Design review of the part built by this model. Coordinates are the model's own, in mm. Coordinates: 2 decimals unless noted, no trailing zeros. Write each loop counter-clockwise with the first axis right and the second up, starting at its lowest first coordinate (ties: lowest second). Pieces come first, ordered by that corner, then holes.
```python
from build123d import *

# Parameters (mm, degrees)
EXTRUDE_1_DEPTH = 10


with BuildPart() as part:
    # ｽｹｯﾁ1 → ﾎﾞｽ - 押し出し1 (new body)
    with BuildSketch(Plane(origin=(0, 0, 0), x_dir=(1, 0, 0), z_dir=(0, 1, 0))):
        with BuildLine():
            ThreePointArc((9.1, 0), (10.6, 1.5), (12.1, 0))
            Line((12.1, 0), (25, 0))
            Line((25, 0), (25, 25))
            Line((25, 25), (-25, 25))
            Line((-25, 25), (-25, 0))
            Line((-25, 0), (-15.5, 0))
            ThreePointArc((-15.5, 0), (-14, 1.5), (-12.5, 0))
            Line((-12.5, 0), (0, 0))
            Line((0, 0), (9.1, 0))
        make_face()
        with BuildLine():
            Line((25, 0), (12.1, 0))
            ThreePointArc((12.1, 0), (10.6, -1.5), (9.1, 0))
            Line((9.1, 0), (0, 0))
            Line((0, 0), (-12.5, 0))
            ThreePointArc((-12.5, 0), (-14, -1.5), (-15.5, 0))
            Line((-15.5, 0), (-25, 0))
            Line((-25, 0), (-25, -25))
            Line((-25, -25), (25, -25))
            Line((25, -25), (25, 0))
        make_face()
    extrude(amount=EXTRUDE_1_DEPTH)


solid = part.part
```
(1) Insertion check: pin 1 Ø6 at (x, z) = (20, -10.5) entering from -Y; pin 2 Ø2.5 at (x, z) = (-14, 0) entering from +Y. Each pin has a flat end and moves straight along its axis. Give the tip position at first contact, or say it passes through.
(2) Consider section A-A (x = 10.6). Give the boundary of the cut face in (y, z).
(3) Mouldability with a two-part tool opening along Z and no side actions: class faces 1 (the cylindrical face through (11.986, 4.93, -0.575)), 2 (the flat face through (0, 5, 25)), 3 (the flat face through (0, 5, -25)), 4 (the flat face through (0, 0, 0)) as +Z half, -Z half, draft (parallel to the pull), parting line (faces both ways), or undercut.
(4) Consider section B-B (z = 0). Give the boundary of the cut face in (x, y).
(5) Wall thickness on line 1 (Z direction, x = -14, y = 8.25); line 2 (X direction, y = 3.5, z = -1); line 3 (Z direction, x = 11.5, y = 1.5): over which ranges is each line inside the solid? List them lowest first.
Results:
1. pin 1: stops at y = 0
1. pin 2: passes through
2. outline: (0, -25) - (10, -25) - (10, -1.5) - (0, -1.5) - close; (0, 1.5) - (10, 1.5) - (10, 25) - (0, 25) - close
3. face 1: undercut
3. face 2: +Z half
3. face 3: -Z half
3. face 4: draft
4. outline: (-25, 0) - (-15.5, 0) - (-15.5, 10) - (-25, 10) - close; (-12.5, 0) - (9.1, 0) - (9.1, 10) - (-12.5, 10) - close; (12.1, 0) - (25, 0) - (25, 10) - (12.1, 10) - close
5. line 1: z = -25 to -1.5, 1.5 to 25
5. line 2: x = -25 to -15.12, -12.88 to 9.48, 11.72 to 25
5. line 3: z = -25 to -1.2, 1.2 to 25
